Geometry check sheet. Reference: the model listing, model coordinates, mm. A direction names the side the tool comes from. Round coordinates to 2 decimals unless told otherwise and drop trailing zeros. Loops run counter-clockwise (first coordinate to the right, second up) from the corner with the lowest first, then second, coordinate; pieces in that order, holes last. Notation, with made-up numbers: M 80,53.25 L 103,53.25 A12 cw 103,67.25 Z; hole C 2.5,-34 d1. An arc over 180 degrees is marked long. Use one line per item in the form item = value. Start each with the question number.
1. Draft check along Y on faces 4 (the flat face through (-1, -25, -12.7)), 5 (the flat face through (-1, -50.8, -6)), 6 (the cylindrical face through (-40.48, -28.42, -6.26)). Enter one of: pulls with the +Y half, pulls with the -Y half, needs draft (parallel to the pull), parting line crosses it, or undercut.
2. Cross-section at C-C (y = -9). Record the boundary of the cut face in (x, z).
3. Material ranges on line 1 (X direction, y = -25, z = -8); line 2 (Z direction, x = -0.5, y = -13); line 3 (X direction, y = -7, z = 16), recorded low to high.
4. Go/stop test with flat-tipped pins: pin 1 (12 mm diameter, centred on y = -12, z = 20, fed in from +X); pin 2 (19 mm diameter, centred on x = -53.5, y = -18.5, fed in from +Z); pin 3 (5 mm diameter, centred on y = -17.5, z = 32, fed in from -X). Record where each tip stops, or that it passes through.
5. Cross-section at D-D (y = -19). Record the boundary of the cut face in (x, z), then the cut area to 3 significant figures.
6. Cross-section at A-A (y = -25.4). Record the boundary of the cut face in (x, z), then the cut area to 3 significant figures.
7. Set-up check for faces 1 (the cylindrical face through (0.63, -15.87, 56.89)), 2 (the flat face through (-56, -25, 0)), 3 (the flat face through (28.448, -25, 14)): record each of +Z, -Z, +X, -X, +Y, -Y from which the full face is reachable in a straight line by a thin tool's end or side.
8. Cross-section at B-B (x = 53). Record the boundary of the cut face in (y, z), then the cut area to 3 significant figures.
```python
from build123d import *

# Parameters (mm, degrees)
F0_R     = 14.224
F1_DEPTH = 50.8
F2_R     = 7.874
F3_DEPTH = 25.4
F5_DEPTH = 76.2


# Not quite as in the source:
# - a feature names something its author has since deleted; it is built from what else it names


with BuildPart() as f1:
    # F0 (on Front) → F1 (new body)
    with BuildSketch(Plane.XZ):
        with BuildLine():
            Line((28.448, 0), (28.448, 28.448))
            ThreePointArc((28.448, 28.448), (0, 56.896), (-28.448, 28.448))
            Line((-28.448, 28.448), (-28.448, 0))
            Line((-28.448, 0), (-66.548, 0))
            Line((-66.548, 0), (-66.548, -12.7))
            Line((-66.548, -12.7), (67.056, -12.7))
            Line((67.056, -12.7), (67.056, 0))
            Line((67.056, 0), (28.448, 0))
        make_face()
        with Locations((0, 28.448)):
            Circle(F0_R, mode=Mode.SUBTRACT)
    extrude(amount=F1_DEPTH)

    # F2 (on face) → F3 (cut)
    with BuildSketch(Plane.XY):
        with Locations((-47.752, -25.4)):
            Circle(F2_R)
        with Locations((47.752, -25.4)):
            Circle(F2_R)
    extrude(amount=-F3_DEPTH, mode=Mode.SUBTRACT)

    # F4 (on face) → F5 (cut)
    with BuildSketch(Plane.YZ.offset(28.448)):
        Polygon((-50.8, 28.448), (-50.8, 3.048), (-41.5551560496, 28.448), align=None)
        Polygon((-50.8, 28.448), (-41.5551560496, 28.448), (-26.8481459022, 68.8551782879), (-50.8, 64.0367791057), align=None)
    extrude(amount=-F5_DEPTH, mode=Mode.SUBTRACT)


solid = f1.part
```
Reported:
q1.face_4 = needs draft
q1.face_5 = pulls with the -Y half
q1.face_6 = undercut
q2.outline = M -66.55,-12.7 L 67.06,-12.7 L 67.06,0 L 28.45,0 L 28.45,28.45 A28.45 ccw -28.45,28.45 L -28.45,0 L -66.55,0 Z; hole C 0,28.45 d28.45
q3.line_1 = -66.55 to -55.62, -39.89 to 39.89, 55.62 to 67.06
q3.line_2 = -12.7 to 14.23, 42.66 to 56.89
q3.line_3 = -28.45 to -6.88, 6.88 to 28.45
q4.pin_1 = 28.45
q4.pin_2 = 0
q4.pin_3 = -28.43
q5.outline = M -66.55,-12.7 L -52.34,-12.7 L -52.34,0 L -66.55,0 Z; M -43.17,-12.7 L 43.17,-12.7 L 43.17,0 L 28.45,0 L 28.45,28.45 A28.45 ccw -28.45,28.45 L -28.45,0 L -43.17,0 Z; M 52.34,-12.7 L 67.06,-12.7 L 67.06,0 L 52.34,0 Z; hole C 0,28.45 d28.45
q5.area = 3,720 mm²
q6.outline = M -66.55,-12.7 L -55.63,-12.7 L -55.63,0 L -66.55,0 Z; M -39.88,-12.7 L 39.88,-12.7 L 39.88,0 L 28.45,0 L 28.45,28.45 A28.45 ccw -28.45,28.45 L -28.45,0 L -39.88,0 Z; M 55.63,-12.7 L 67.06,-12.7 L 67.06,0 L 55.63,0 Z; hole C 0,28.45 d28.45
q6.area = 3,550 mm²
q7.face_1 = +Z, +Y, -Y
q7.face_2 = +Z, -X, +Y, -Y
q7.face_3 = +Z, +X, +Y, -Y
q8.outline = M -50.8,-12.7 L -31.27,-12.7 L -31.27,0 L -50.8,0 Z; M -19.53,-12.7 L 0,-12.7 L 0,0 L -19.53,0 Z
q8.area = 496 mm²
